Geometry check sheet. Reference: the model listing, model coordinates, mm. Face numbers are marked on the shaded views. A direction names the side the tool comes from. Round coordinates to 2 decimals unless told otherwise and drop trailing zeros. Order: outer loops, then holes, each group sorted by start corner. A loop starts at its lowest first (then second) coordinate and runs counter-clockwise, first axis right, second up. Notation, with made-up numbers: (78.5, -30.5) - (113.5, -30.5) arc R34 ccw to (113.5, 2.5) - close; hole circle Ø3 at (33, 28). An arc over 180 degrees is marked (long way). Return JSON: item names as keys, results as strings. Group by question number.
Q1. Draft check along X on the marked faces 1, 2 and 3. Enter one of: pulls with the +X half, pulls with the -X half, needs draft (parallel to the pull), parting line crosses it, or undercut.
Q2. Tool access check on the marked faces 4 and 5. Record the directions out of +Z, -Z, +X, -X, +Y, -Y that give a thin tool (end or side, any length) a straight path to the whole face; none if there is none.
Q3. Material ranges on line 1 along Y through (x, z) = (-44.85, 67.5); line 2 along Y through (x, z) = (-32.5, 43); line 3 along Z through (x, y) = (36, 0.5), recorded low to high.
Q4. Sectioned sample at D-D, the plane z = 29.5. Record the cut outline in (x, y).
Q5. Sectioned sample at C-C, the plane x = 44.85. Record the cut outline in (y, z).
Q6. Sectioned sample at A-A, the plane y = 0. Record the cut outline in (x, z).
Q7. Gauge pin test, flat ends, axial feed: pin 1 Ø6 at (x, z) = (40, 17) entering from -Y; pin 2 Ø10 at (y, z) = (-19, 49.5) entering from -X; pin 3 Ø12 at (x, y) = (-41, -31) entering from -Z; pin 4 Ø6.5 at (x, z) = (-37, 67.5) entering from +Y. Record the tip position at first contact, or that the pin passes through.
```python
from build123d import *

# Parameters (mm, degrees)
ESQUISSE1_R        = 50
ESQUISSE1_R_2      = 35
BOSS_EXTRU_2_DEPTH = 10
ESQUISSE4_R        = 7.4
BOSS_EXTRU_3_DEPTH = 70
ESQUISSE5_W        = 20
ESQUISSE5_H        = 14.8
ESQUISSE5_R        = 2.588125741
ESQUISSE5_R_2      = 3.00370922
BOSS_EXTRU_4_DEPTH = 6


with BuildPart() as part:
    # Esquisse1 → Boss.-Extru.2 (new body)
    with BuildSketch(Plane.XY):
        Circle(ESQUISSE1_R)
        Circle(ESQUISSE1_R_2, mode=Mode.SUBTRACT)
    extrude(amount=BOSS_EXTRU_2_DEPTH)

    # Esquisse4 → Boss.-Extru.3 (add)
    with BuildSketch(Plane.XY):
        with Locations((-31.85, -28)):
            Circle(ESQUISSE4_R)
        with Locations((31.85, -28)):
            Circle(ESQUISSE4_R)
    extrude(amount=BOSS_EXTRU_3_DEPTH)

    # Esquisse5 → Boss.-Extru.4 (add)
    # profile 1 of 2: a face of its own
    with BuildSketch(Plane.XY.offset(70)):
        with Locations((-41.85, -28)):
            Rectangle(ESQUISSE5_W, ESQUISSE5_H)
        with Locations((-44.85, -28)):
            Circle(ESQUISSE5_R, mode=Mode.SUBTRACT)
    # profile 2 of 2: a face of its own
    with BuildSketch(Plane.XY.offset(70)):
        with Locations((41.85, -28)):
            Rectangle(ESQUISSE5_W, ESQUISSE5_H)
        with Locations((44.85, -28)):
            Circle(ESQUISSE5_R_2, mode=Mode.SUBTRACT)
    extrude(amount=-BOSS_EXTRU_4_DEPTH)


solid = part.part
```
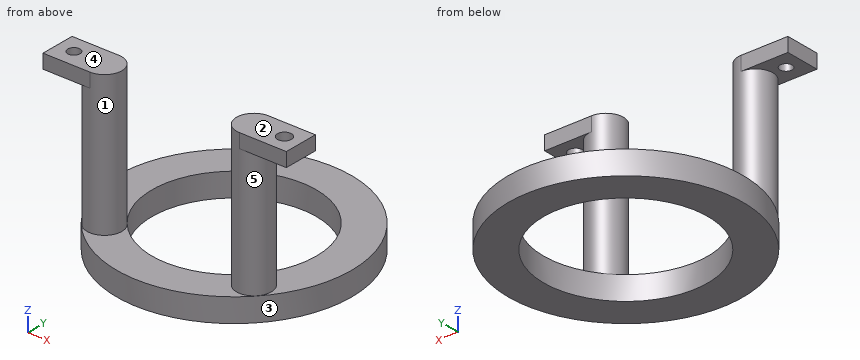
Reply:
{
 "1": {"face 1": "undercut", "face 2": "needs draft", "face 3": "parting line crosses it"},
 "2": {"face 4": "+Z, +X, -X, +Y, -Y", "face 5": "none"},
 "3": {"line 1": "-35.4 to -30.59, -25.41 to -20.6", "line 2": "-35.37 to -20.63", "line 3": "0 to 10"},
 "4": {"outline": "circle Ø14.8 at (-31.85, -28); circle Ø14.8 at (31.85, -28)"},
 "5": {"outline": "(-35.4, 64) - (-31, 64) - (-31, 70) - (-35.4, 70) - close; (-25, 64) - (-20.6, 64) - (-20.6, 70) - (-25, 70) - close; (-22.1, 0) - (22.1, 0) - (22.1, 10) - (-22.1, 10) - close"},
 "6": {"outline": "(-50, 0) - (-35, 0) - (-35, 10) - (-50, 10) - close; (35, 0) - (50, 0) - (50, 10) - (35, 10) - close"},
 "7": {"pin 1": "y = -33.31", "pin 2": "x = -38.08", "pin 3": "z = 0", "pin 4": "y = -20.6"}
}
